```python
from build123d import *

# Parameters (mm, degrees)
ESQUISSE1_R        = 1.4
BOSS_EXTRU_1_DEPTH = 9
ESQUISSE2_R        = 3.25
BOSS_EXTRU_2_DEPTH = 1
CONG_1_R           = 1
CONG_2_R           = 0.25


with BuildPart() as part:
    # Esquisse1 → Boss.-Extru.1 (new body)
    with BuildSketch(Plane.XY):
        with Locations((-28.068256791, 21.884700983)):
            Circle(ESQUISSE1_R)
    extrude(amount=BOSS_EXTRU_1_DEPTH)

    # Esquisse2 → Boss.-Extru.2 (add)
    with BuildSketch(Plane.XY.offset(9)):
        with Locations((-28.068256791, 21.884700983)):
            Circle(ESQUISSE2_R)
    extrude(amount=BOSS_EXTRU_2_DEPTH)

    # Congé1
    cong_1_edges = [part.edges().sort_by_distance(p)[0] for p in [
        (-31.318256791, 21.884700983, 10),
    ]]
    fillet(cong_1_edges, radius=CONG_1_R - 0.0001)  # a hair under: the kernel refuses the full size

    # Congé2
    cong_2_edges = [part.edges().sort_by_distance(p)[0] for p in [
        (-29.468256791, 21.884700983, 0),
    ]]
    fillet(cong_2_edges, radius=CONG_2_R)


solid = part.part
```
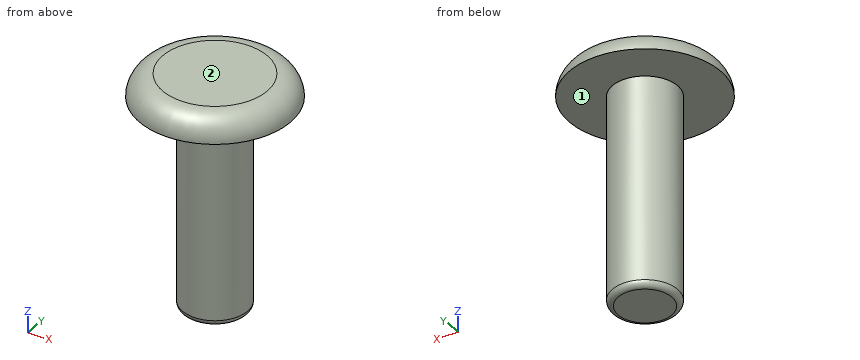
Can you work these out from the model? Positions are in its coordinate system, mm. Face numbers are marked on the shaded views. A direction names the side the tool comes from. Coordinates: 2 decimals unless noted, no trailing zeros. Loops run counter-clockwise (first coordinate to the right, second up) from the corner with the lowest first, then second, coordinate; pieces in that order, holes last.
1) Imagine slicing it at A-A on z = 6.25. List the corners of the cut face in (x, y) for me, plus the area to 3 significant figures.
2) Which directions (+Z, -Z, +X, -X, +Y, -Y) give clear straight access to the entire face, cutting with the end or side of a thin tool? Please do the marked faces 1 and 2.
3) I need wall thicknesses on probe 1 along Z at (x, y) = (-26, 22); probe 2 along Y at (x, z) = (-28, 7.25); probe 3 along Y at (x, z) = (-30.5, 9.25). Which ranges of each line are inside material? Lowest first, please.
4) For pin 1 (1 mm diameter, centred on y = 23.5, z = 7.5, fed in from +X); pin 2 (2 mm diameter, centred on y = 24, z = 1, fed in from -X), each with a flat end and sliding along its axis, tell me the tip position at first contact or that it passes through.
Completed:
1. outline: circle Ø2.8 at (-28.07, 21.88)
1. area: 6.16 mm2
2. face 1: -Z
2. face 2: +Z, +X, -X, +Y, -Y
3. probe 1: z = 9 to 10
3. probe 2: y = 20.49 to 23.28
3. probe 3: y = 19.78 to 23.99
4. pin 1: stops at x = -27.22
4. pin 2: stops at x = -28.91
